Model file for the job. Use its own axes, mm. A direction names the side the tool comes from. Round coordinates to 2 decimals unless told otherwise and drop trailing zeros. Order: outer loops, then holes, each group sorted by start corner. A loop starts at its lowest first (then second) coordinate and runs counter-clockwise, first axis right, second up. Notation, with made-up numbers: (-2, 45) - (12, 45) arc R12 ccw to (12, 53) - close; hole circle Ø4 at (71, -7). An arc over 180 degrees is marked (long way). Put each result on its own line as item: value. Start each with the question number.
Item 1: Which spindle directions (+Z, -Z, +X, -X, +Y, -Y) get a long thin tool onto all of the face, cutting with end or side? Do faces 4 (the face through (8, -20, 15)), 5 (the face through (29.35, -25.07, 57.6)), 6 (the face through (49.3, -30, 35.5)). Say none if no direction does.
Item 2: Saw through at A-A on x = 40. List the corners of the cut face in (y, z).
Item 3: Pin check, flat tips, straight feed: pin 1 Ø5 at (y, z) = (-13.5, 57.5) entering from -X; pin 2 Ø1.2 at (x, z) = (31.5, 56.5) entering from -Y; pin 3 Ø5 at (y, z) = (-26.5, 6.5) entering from -X. Stop position of each tip, or through.
Item 4: Mould opens along X. For faces 1 (the face through (9, -25, 20)), 2 (the face through (19.43, -24.93, 19.4)), 3 (the face through (74.619, -15.21, 8.085)) say: pulls with the +X half, pulls with the -X half, needs draft (parallel to the pull), parting line crosses it, or undercut.
Item 5: Saw through at D-D on z = 30. List the corners of the cut face in (x, y), plus the area to 3 significant figures.
Item 6: Saw through at B-B on z = 10. List the corners of the cut face in (x, y), plus the area to 3 significant figures.
Item 7: Saw through at C-C on y = -3.5. List the corners of the cut face in (x, z), plus the area to 3 significant figures.
Item 8: Probe probe 1 along Z at (x, y) = (40, -18.25); probe 2 along X at (y, z) = (-20.5, 56.5); probe 3 along Z at (x, y) = (74.5, -25.25). List the from-to ranges inside material, lowest first.
```python
from build123d import *

# Parameters (mm, degrees)
F0_W      = 100
F0_H      = 70
F1_DEPTH  = 30
F3_DEPTH  = 9
F4_W      = 20
F4_H      = 20
F5_DEPTH  = 10
F6_R      = 5
F7_DEPTH  = 25
F8_R      = 2
F9_DEPTH  = 10
F10_R     = 5
F11_DEPTH = 41.45141
F12_SIZE  = 5
F13_R     = 2


with BuildPart() as f1:
    # F0 (on Front) → F1 (new body)
    with BuildSketch(Plane.XZ):
        with Locations((50, 35)):
            Rectangle(F0_W, F0_H)
    extrude(amount=F1_DEPTH)

    # F2 (on face) → F3 (cut)
    with BuildSketch(Plane.XZ.offset(30)):
        with BuildLine():
            Line((85.000001, 70), (75, 70))
            Line((75, 70), (75, 50))
            Line((75, 50), (50, 50))
            ThreePointArc((50, 50), (45, 45), (50, 39.999999))
            Line((50, 39.999999), (77.928933, 39.999999))
            Line((77.928933, 39.999999), (100, 17.928932))
            Line((100, 17.928932), (100, 32.07107))
            Line((100, 32.07107), (85.000001, 47.071069))
            Line((85.000001, 47.071069), (85.000001, 70))
        make_face()
    extrude(amount=-F3_DEPTH, mode=Mode.SUBTRACT)

    # F4 (on face) → F5 (cut)
    with BuildSketch(Plane.XZ.offset(30)):
        with Locations((10, 10)):
            Rectangle(F4_W, F4_H)
    extrude(amount=-F5_DEPTH, mode=Mode.SUBTRACT)

    # F6 (on face) → F7 (cut)
    with BuildSketch(Plane.XZ.offset(20)):
        with Locations((10, 10)):
            Circle(F6_R)
    extrude(amount=-F7_DEPTH, mode=Mode.SUBTRACT)

    # F8 (on face) → F9 (cut)
    with BuildSketch(Plane.XZ.offset(30)):
        with Locations((20, 62.5)):
            Circle(F8_R)
        with Locations((9.174682, 56.25)):
            Circle(F8_R)
        with Locations((9.174682, 43.75)):
            Circle(F8_R)
        with Locations((20, 37.5)):
            Circle(F8_R)
        with Locations((30.825318, 43.75)):
            Circle(F8_R)
        with Locations((30.825318, 56.25)):
            Circle(F8_R)
    extrude(amount=-F9_DEPTH, mode=Mode.SUBTRACT)

    # F10 (on face) → F11 (cut)
    with BuildSketch(Plane.XZ.offset(30)):
        with Locations((40, 10)):
            Circle(F10_R)
        with Locations((55, 10)):
            Circle(F10_R)
        with Locations((70, 10)):
            Circle(F10_R)
        with Locations((50, 30)):
            Circle(F10_R)
    extrude(amount=-F11_DEPTH, mode=Mode.SUBTRACT)

    # F12
    f12_edges = [f1.edges().sort_by_distance(p)[0] for p in [
        (100, -15, 0),
    ]]
    chamfer(f12_edges, length=F12_SIZE)

    # F13
    f13_edges = [f1.edges().sort_by_distance(p)[0] for p in [
        (20, -25, 20),
    ]]
    fillet(f13_edges, radius=F13_R)


solid = f1.part
```
Results found:
1. face 4: -Z, -X, -Y
1. face 5: -Y
1. face 6: +Z, -Z, +X, -X, -Y
2. outline: (-30, 0) - (0, 0) - (0, 5) - (-30, 5) - close; (-30, 15) - (0, 15) - (0, 70) - (-30, 70) - close
3. pin 1: stops at x = 0
3. pin 2: stops at y = -20
3. pin 3: stops at x = 20
4. face 1: needs draft
4. face 2: pulls with the -X half
4. face 3: undercut
5. outline: (0, -30) - (45, -30) - (45, 0) - (0, 0) - close; (55, -30) - (87.93, -30) - (87.93, -21) - (100, -21) - (100, 0) - (55, 0) - close
5. area: 2,590 mm²
6. outline: (0, -20) - (5, -20) - (5, 0) - (0, 0) - close; (15, -20) - (20, -20) - (20, -30) - (35, -30) - (35, 0) - (15, 0) - close; (45, -30) - (50, -30) - (50, 0) - (45, 0) - close; (60, -30) - (65, -30) - (65, 0) - (60, 0) - close; (75, -30) - (100, -30) - (100, 0) - (75, 0) - close
6. area: 1,700 mm²
7. outline: (0, 0) - (95, 0) - (100, 5) - (100, 70) - (0, 70) - close; hole circle Ø10 at (10, 10); hole circle Ø10 at (40, 10); hole circle Ø10 at (50, 30); hole circle Ø10 at (55, 10); hole circle Ø10 at (70, 10)
7. area: 6,590 mm²
8. probe 1: z = 0 to 5, 15 to 70
8. probe 2: x = 0 to 7.19, 11.16 to 28.84, 32.81 to 100
8. probe 3: z = 0 to 7.82, 12.18 to 40, 50 to 70
